Work out the finished part from the listing and answer in its coordinate system (mm). Face numbers are marked on the shaded views. A direction names the side the tool comes from. Give positions to 0.01 mm unless a question says otherwise; leave off trailing zeros. Loops run counter-clockwise (first coordinate to the right, second up) from the corner with the lowest first, then second, coordinate; pieces in that order, holes last.
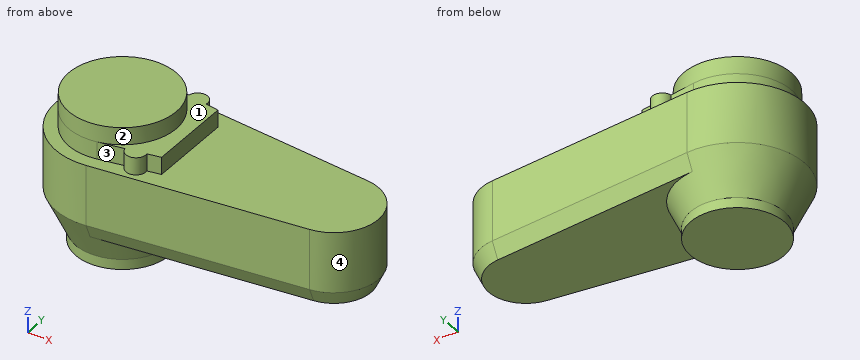
Autodesk Inventor part; units mm, degrees
ref_plane "Work Plane1" through (0, 0, 105) normal (0, 0, -1) x (-1, 0, 0)
ref_plane "Work Plane2" through (0, 0, 74) normal (0, 0, -1) x (-1, 0, 0)
ref_plane "YZ Plane" through (0, 0, 0) normal (1, 0, 0) x (0, 1, 0)
sketch "Sketch1" plane through (0, 0, 0) normal (0, 0, 1) x (1, 0, 0)
  circle A0 centre (0, 0) radius 94
  dimension "d0" = 188
extrude "Extrusion1" add sketch "Sketch1" along normal blind 20.292
ref_plane "Work Plane1" through (0, 0, 105) normal (0, 0, -1) x (-1, 0, 0)
sketch "Sketch2" plane through (0, 0, 105) normal (0, 0, -1) x (-1, 0, 0)
  circle A0 centre (0, 0) radius 133.5
  dimension "d4" = 267
loft "Loft1" add profiles "Sketch2" section 2 edges at (-94, 0, 20.292)
sketch "Sketch3" plane through (0, 0, 105) normal (0, 0, 1) x (1, 0, 0)
  circle A0 centre (0, 0) radius 133.5 construction
  circle A1 centre (425, 0) radius 89 construction
  line L0 (13.9782, 132.7662) -> (434.3188, 88.5108)
  circle A2 centre (0, 0) radius 133.5
  line L1 (13.9782, -132.7662) -> (434.3188, -88.5108)
  arc A3 (13.9782, 132.7662) -> (13.9782, -132.7662) centre (0, 0) ccw
  arc A4 (434.3188, -88.5108) -> (434.3188, 88.5108) centre (425, 0) ccw
  dimension "d9" = 178
  dimension "d10" = 425
extrude "Extrusion2" add sketch "Sketch3" along normal blind 121
ref_plane "Work Plane2" through (0, 0, 74) normal (0, 0, -1) x (-1, 0, 0)
sketch "Sketch4" plane through (0, 0, 74) normal (0, 0, -1) x (-1, 0, 0)
  arc A0 (-434.3188, 88.5108) -> (-434.3188, -88.5108) centre (-425, 0) ccw construction
  circle A1 centre (-425, 0) radius 74.544 construction
  circle A2 centre (0, 0) radius 119.044 construction
  line L0 (-12.4646, -118.3896) -> (-432.8052, -74.1342)
  line L1 (-12.4646, 118.3896) -> (-432.8052, 74.1342)
  line L2 (-13.9782, -132.7662) -> (-434.3188, -88.5108)
  line L3 (-434.3188, 88.5108) -> (-13.9782, 132.7662)
  arc A3 (-12.4646, -118.3896) -> (-12.4646, 118.3896) centre (0, 0) ccw
  arc A4 (-432.8052, 74.1342) -> (-432.8052, -74.1342) centre (-425, 0) ccw
  dimension "d14" = 149.088
  dimension "d15" = 238.088
loft "Loft2" add profiles "Sketch4" section 2 edges at (133.5, 0, 105) (224.1485, 110.6385, 105) (514, 0, 105) (224.1485, -110.6385, 105)
sketch "Sketch7" plane through (0, 0, 226) normal (0, 0, 1) x (1, 0, 0)
  circle A0 centre (0, 0) radius 108 construction
  line L0 (135, 85.862) -> (135, -85.862)
  line L1 (135, -85.862) -> (135, 85.862) construction
  line L2 (18.7539, 106.3592) -> (135, 85.862) construction
  line L3 (135, -85.862) -> (18.7539, -106.3592) construction
  circle A1 centre (89, 93.973) radius 20 construction
  circle A2 centre (89, -93.973) radius 20 construction
  line L4 (135, 85.862) -> (108.6962, 90.5001)
  line L5 (135, -85.862) -> (108.6962, -90.5001)
  arc A3 (69.3038, -97.446) -> (108.6962, -90.5001) centre (89, -93.973) ccw
  arc A4 (108.6962, 90.5001) -> (69.3038, 97.446) centre (89, 93.973) ccw
  line L6 (69.3038, 97.446) -> (18.7539, 106.3592)
  line L7 (69.3038, -97.446) -> (18.7539, -106.3592)
  arc A5 (18.7539, 106.3592) -> (18.7539, -106.3592) centre (0, 0) ccw
  point P0 (135, 0)
  dimension "d33" = 40
  dimension "d30" = 216
  dimension "d31" = 171.724
  dimension "d32" = 135
  dimension "d34" = 89
extrude "Extrusion5" add sketch "Sketch7" along normal blind 34.5
sketch "Sketch8" plane through (0, 0, 260.5) normal (0, 0, 1) x (1, 0, 0)
  circle A0 centre (0, 0) radius 108
  arc A1 (18.7539, 106.3592) -> (18.7539, -106.3592) centre (0, 0) ccw construction
  point P0 (-108, 0)
extrude "Extrusion6" add sketch "Sketch8" along normal blind 34.5
properties part number "1"
Q1. Given pin 1 (2 mm diameter, centred on x = 159, y = -61.5, fed in from -Z); pin 2 (1 mm diameter, centred on x = 421.5, z = 164, fed in from -Y); pin 3 (10 mm diameter, centred on y = -36.5, z = 232.5, fed in from +X), each flat-ended and moving along its own axis, determine where each tip first touches the part or whether it passes through.
Q2. Which of the six approach directions +Z, -Z, +X, -X, +Y, -Y give full straight-line access (tool end or side, diameter ignored) to the marked faces 1, 2, 3 and 4?
Q3. Section A-A on x = 0 is taken. Give the vertices of the cut face in (y, z), plus the area to 3 significant figures.
Q4. Section B-B on z = 38 is taken. Give the vertices of the cut face in (x, y), plus the area to 3 significant figures.
Q5. Consider line 1 along Z through (x, y) = (374.5, 63.5); line 2 along Y through (x, z) = (-0.5, 117.5); line 3 along Y through (x, z) = (24, 111). Determine where each line is inside the solid, lowest interval first.
Q6. Section C-C on z = 202.5 is taken. Give the vertices of the cut face in (x, y), plus the area to 3 significant figures.
Check result:
1. pin 1: stops at z = 74
1. pin 2: stops at y = -89.91
1. pin 3: stops at x = 135
2. face 1: +Z, +X
2. face 2: +Z
2. face 3: +Z, -Y
2. face 4: +Z, -Z, +X
3. outline: (-133.5, 105) - (-94, 20.29) - (-94, 0) - (94, 0) - (94, 20.29) - (133.5, 105) - (133.5, 226) - (108, 226) - (108, 295) - (-108, 295) - (-108, 226) - (-133.5, 226) - close
3. area: 70,300 mm2
4. outline: circle Ø204.51 at (0, 0)
4. area: 32,900 mm2
5. line 1: z = 74 to 226
5. line 2: y = -133.5 to 133.5
5. line 3: y = -131.71 to 131.71
6. outline: (13.98, -132.77) - (434.32, -88.51) arc R89 ccw to (434.32, 88.51) - (13.98, 132.77) arc R133.5 ccw (long way) to start
6. area: 136,000 mm2
